Read the model definition and answer for the solid it produces. Units are mm, in the model's axes. A direction names the side the tool comes from. Coordinates: 2 decimals unless noted, no trailing zeros. Loops run counter-clockwise (first coordinate to the right, second up) from the corner with the lowest first, then second, coordinate; pieces in that order, holes last.
Q1. The mould has two halves that part along X. Classify faces 5 (the face through (-1, 27, 2)), 6 (the face through (-41, 33, 1)), 7 (the face through (54.1, 31.64, 1.01)), 8 (the face through (15.5, 74.93, 0.99)): pulls with the +X half, pulls with the -X half, needs draft (parallel to the pull), parting line crosses it, or undercut.
Q2. Which of the six approach directions +Z, -Z, +X, -X, +Y, -Y give full straight-line access (tool end or side, diameter ignored) to faces 1 (the face through (44, 33, 1)), 2 (the face through (26, 66, 1)), 3 (the face through (24.1, 38.36, 0.99)), 4 (the face through (-54.14, 31.6, 1.01))?
Q3. Section B-B (y = 26.5) is taken. Give the vertices of the cut face in (x, z).
Q4. Section D-D (z = 1.25) is taken. Count the separate pieces of the cut face and the enclosed holes in it, then the cut area to 3 significant figures.
Q5. Section A-A (y = 45.5) is taken. Give the vertices of the cut face in (x, z), then the cut area to 3 significant figures.
Q6. Section C-C (x = -17.5) is taken. Give the vertices of the cut face in (y, z), then the cut area to 3 significant figures.
Q7. Flat-ended cylindrical pins translate along their axes: P1, Ø1, axis at y = 80, z = 0.5, coming from the +X side; P2, Ø1.9, axis at x = 38, y = 79, coming from the +Z side; P3, Ø1, axis at x = 19, z = 1, coming from the +Y side; P4, Ø0.6, axis at x = -46.5, z = 1.5, coming from the +Y side. Find the tip coordinate at first contact, or state that the pin passes through.
Q8. Straight lines are drawn through the part: line 1 (X direction, y = 79, z = 1.2); line 2 (Y direction, x = 38, z = 1.55); line 3 (Y direction, x = 50.5, z = 0.65). For each, find the intervals that lie inside material, in ascending order.
from build123d import *

# Parameters (mm, degrees)
SKETCH_1_W      = 110
SKETCH_1_H      = 65
EXTRUDE_1_DEPTH = 2
FILLET_1_R      = 3
SKETCH_2_R      = 3
EXTRUDE_2_DEPTH = 2
FILLET_5_R      = 3
FILLET_6_R      = 5
SKETCH_4_W      = 10
SKETCH_4_H      = 5
EXTRUDE_4_DEPTH = 2
FILLET_7_R      = 2.5
SKETCH_5_W      = 16
SKETCH_5_H      = 45
SKETCH_5_R      = 1.2
EXTRUDE_5_DEPTH = 2
SKETCH_6_W      = 10
SKETCH_6_H      = 5
SKETCH_6_W_2    = 5
SKETCH_6_H_2    = 10
EXTRUDE_6_DEPTH = 2
FILLET_8_R      = 2.5
FILLET_9_R      = 2


with BuildPart() as part:
    # Sketch 1 → Extrude 1 (new body)
    with BuildSketch(Plane.XY):
        Rectangle(SKETCH_1_W, SKETCH_1_H)
        with BuildLine():
            Line((-49.5, 24.75), (-46.5, 24.75))
            ThreePointArc((-46.5, 24.75), (-44.75, 26.5), (-46.5, 28.25))
            Line((-46.5, 28.25), (-49.5, 28.25))
            ThreePointArc((-49.5, 28.25), (-51.25, 26.5), (-49.5, 24.75))
        make_face(mode=Mode.SUBTRACT)
        with BuildLine():
            Line((-46.5, -20.25), (-49.5, -20.25))
            ThreePointArc((-49.5, -20.25), (-51.25, -18.5), (-49.5, -16.75))
            Line((-49.5, -16.75), (-46.5, -16.75))
            ThreePointArc((-46.5, -16.75), (-44.75, -18.5), (-46.5, -20.25))
        make_face(mode=Mode.SUBTRACT)
        with BuildLine():
            Line((46.5, -20.25), (49.5, -20.25))
            ThreePointArc((49.5, -20.25), (51.25, -18.5), (49.5, -16.75))
            Line((49.5, -16.75), (46.5, -16.75))
            ThreePointArc((46.5, -16.75), (44.75, -18.5), (46.5, -20.25))
        make_face(mode=Mode.SUBTRACT)
        with BuildLine():
            Line((46.5, 28.25), (49.5, 28.25))
            ThreePointArc((49.5, 28.25), (51.25, 26.5), (49.5, 24.75))
            Line((49.5, 24.75), (46.5, 24.75))
            ThreePointArc((46.5, 24.75), (44.75, 26.5), (46.5, 28.25))
        make_face(mode=Mode.SUBTRACT)
    extrude(amount=EXTRUDE_1_DEPTH)

    # Fillet 1
    fillet_1_edges = [part.edges().sort_by_distance(p)[0] for p in [
        (-55, 32.5, 1),
        (55, 32.5, 1),
        (55, -32.5, 1),
        (-55, -32.5, 1),
    ]]
    fillet(fillet_1_edges, radius=FILLET_1_R)



with BuildPart() as body_2:
    # Sketch 2 → Extrude 2 (new body)
    with BuildSketch(Plane.XY.offset(2)):
        Polygon((-55, 37.5), (25, 37.5), (25, 73.5), (14, 73.5), (14, 85.5), (-44, 85.5), (-44, 73.5), (-55, 73.5), align=None)
        with Locations((14, 67.5)):
            Circle(SKETCH_2_R, mode=Mode.SUBTRACT)
        with BuildLine():
            Line((-45.5, 64.5), (-42.5, 64.5))
            ThreePointArc((-42.5, 64.5), (-39.5, 67.5), (-42.5, 70.5))
            Line((-42.5, 70.5), (-45.5, 70.5))
            ThreePointArc((-45.5, 70.5), (-48.5, 67.5), (-45.5, 64.5))
        make_face(mode=Mode.SUBTRACT)
    extrude(amount=-EXTRUDE_2_DEPTH)

    # Fillet 5
    fillet_5_edges = [body_2.edges().sort_by_distance(p)[0] for p in [
        (25, 37.5, 1),
        (-55, 37.5, 1),
        (-55, 73.5, 1),
        (-44, 85.5, 1),
        (14, 85.5, 1),
        (25, 73.5, 1),
    ]]
    fillet(fillet_5_edges, radius=FILLET_5_R)

    # Fillet 6
    fillet_6_edges = [body_2.edges().sort_by_distance(p)[0] for p in [
        (-44, 73.5, 1),
        (14, 73.5, 1),
    ]]
    fillet(fillet_6_edges, radius=FILLET_6_R)


with BuildPart() as part_1:
    add(part.part)

    add(body_2.part)  # Extrude 4 merges body 2
    # Sketch 4 → Extrude 4 (add)
    with BuildSketch(Plane.XY.offset(2)):
        with Locations((-35, 35)):
            Rectangle(SKETCH_4_W, SKETCH_4_H)
        with Locations((5, 35)):
            Rectangle(SKETCH_4_W, SKETCH_4_H)
    extrude(amount=-EXTRUDE_4_DEPTH)

    # Fillet 7
    fillet_7_edges = [part_1.edges().sort_by_distance(p)[0] for p in [
        (10, 37.5, 1),
        (10, 32.5, 1),
        (0, 37.5, 1),
        (0, 32.5, 1),
        (-30, 37.5, 1),
        (-30, 32.5, 1),
        (-40, 37.5, 1),
        (-40, 32.5, 1),
    ]]
    fillet(fillet_7_edges, radius=FILLET_7_R - 0.0001)  # a hair under: the kernel refuses the full size



with BuildPart() as body_2_2:
    # Sketch 5 → Extrude 5 (new body)
    with BuildSketch(Plane.XY.offset(2)):
        with Locations((38, 60)):
            Rectangle(SKETCH_5_W, SKETCH_5_H)
        with Locations((38, 79)):
            Circle(SKETCH_5_R, mode=Mode.SUBTRACT)
        with BuildLine():
            Line((36.683223365, 42), (36.683223365, 40))
            ThreePointArc((36.683223365, 40), (37.883223365, 38.8), (39.083223365, 40))
            Line((39.083223365, 40), (39.083223365, 42))
            ThreePointArc((39.083223365, 42), (37.883223365, 43.2), (36.683223365, 42))
        make_face(mode=Mode.SUBTRACT)
    extrude(amount=-EXTRUDE_5_DEPTH)


with BuildPart() as part_2:
    add(part_1.part)

    add(body_2_2.part)  # Extrude 6 merges body 2 2
    # Sketch 6 → Extrude 6 (add)
    with BuildSketch(Plane.XY.offset(2)):
        with Locations((38, 35)):
            Rectangle(SKETCH_6_W, SKETCH_6_H)
        with Locations((27.5, 60.5)):
            Rectangle(SKETCH_6_W_2, SKETCH_6_H_2)
    extrude(amount=-EXTRUDE_6_DEPTH)

    # Fillet 8
    fillet_8_edges = [part_2.edges().sort_by_distance(p)[0] for p in [
        (43, 32.5, 1),
        (43, 37.5, 1),
        (33, 32.5, 1),
        (33, 37.5, 1),
        (30, 55.5, 1),
        (25, 55.5, 1),
        (25, 65.5, 1),
        (30, 65.5, 1),
    ]]
    fillet(fillet_8_edges, radius=FILLET_8_R - 0.0001)  # a hair under: the kernel refuses the full size

    # Fillet 9
    fillet_9_edges = [part_2.edges().sort_by_distance(p)[0] for p in [
        (46, 82.5, 1),
        (30, 82.5, 1),
        (46, 37.5, 1),
        (30, 37.5, 1),
    ]]
    fillet(fillet_9_edges, radius=FILLET_9_R)


solid = part_2.part
Numbers:
1. face 5: needs draft
1. face 6: pulls with the -X half
1. face 7: pulls with the +X half
1. face 8: undercut
2. face 1: +Z, -Z, +X
2. face 2: +Z, -Z, +Y
2. face 3: +Z, -Z
2. face 4: +Z, -Z, -X
3. outline: (-55, 0) - (-51.25, 0) - (-51.25, 2) - (-55, 2) - close; (-44.75, 0) - (44.75, 0) - (44.75, 2) - (-44.75, 2) - close; (51.25, 0) - (55, 0) - (55, 2) - (51.25, 2) - close
4. separate pieces: 1
4. enclosed holes: 10
4. area: 11,500 mm2
5. outline: (-55, 0) - (25, 0) - (25, 2) - (-55, 2) - close; (30, 0) - (46, 0) - (46, 2) - (30, 2) - close
5. area: 192 mm2
6. outline: (-32.5, 0) - (32.5, 0) - (32.5, 2) - (-32.5, 2) - close; (37.5, 0) - (85.5, 0) - (85.5, 2) - (37.5, 2) - close
6. area: 226 mm2
7. P1: stops at x = 46
7. P2: passes through
7. P3: stops at y = 73.53
7. P4: stops at y = 74.36
8. line 1: x = -44 to 14, 30 to 36.8, 39.2 to 46
8. line 2: y = -32.5 to 38.81, 43.19 to 77.8, 80.2 to 82.5
8. line 3: y = -32.5 to -19.94, -17.06 to 25.06, 27.94 to 32.5
